```python
from build123d import *

# Parameters (mm, degrees)
BOSS_EXTRUDE1_DEPTH = 9
CUT_EXTRUDE2_REACH  = 95.842
SKETCH5_W           = 20
SKETCH5_H           = 32
SKETCH5_W_2         = 7.75
CUT_EXTRUDE3_DEPTH  = 10
FILLET1_R           = 5
CUT_EXTRUDE4_DEPTH  = 4
CHAMFER1_SIZE       = 9
CHAMFER1_SIZE_2     = 4.196768923
CUT_EXTRUDE5_REACH  = 95.842
SKETCH7_W           = 5
SKETCH7_H           = 33.085129134
SKETCH7_H_2         = 33.745309592


with BuildPart() as part:
    # Sketch1 → Boss-Extrude1 (new body)
    with BuildSketch(Plane(origin=(0, 0, 0), x_dir=(1, 0, 0), z_dir=(0, 1, 0))):
        with BuildLine():
            Line((0, 0), (0, 55))
            Line((0, 55), (75.5, 55))
            Line((75.5, 55), (75.5, 0))
            ThreePointArc((75.5, 0), (37.75, 13.36377481), (0, 0))
        make_face()
    extrude(amount=BOSS_EXTRUDE1_DEPTH)

    # Sketch4 → Cut-Extrude2 (cut, up to next)
    with BuildSketch(Plane(origin=(0, 9, 0), x_dir=(1, 0, 0), z_dir=(0, 1, 0)), mode=Mode.PRIVATE) as cut_extrude2_sk1:
        with BuildLine():
            Line((19.25, 48), (19.25, 23))
            ThreePointArc((19.25, 23), (17.75, 21.5), (16.25, 23))
            Line((16.25, 23), (16.25, 48))
            ThreePointArc((16.25, 48), (17.75, 49.5), (19.25, 48))
        make_face()
    cut_extrude2_tool1 = extrude(cut_extrude2_sk1.sketch, amount=-CUT_EXTRUDE2_REACH, mode=Mode.PRIVATE) & part.part
    # Sketch4 → Cut-Extrude2 (cut, up to next)
    with BuildSketch(Plane(origin=(0, 9, 0), x_dir=(1, 0, 0), z_dir=(0, 1, 0)), mode=Mode.PRIVATE) as cut_extrude2_sk2:
        with BuildLine():
            Line((59.25, 48), (59.25, 23))
            ThreePointArc((59.25, 23), (57.75, 21.5), (56.25, 23))
            Line((56.25, 23), (56.25, 48))
            ThreePointArc((56.25, 48), (57.75, 49.5), (59.25, 48))
        make_face()
    cut_extrude2_tool2 = extrude(cut_extrude2_sk2.sketch, amount=-CUT_EXTRUDE2_REACH, mode=Mode.PRIVATE) & part.part
    add(cut_extrude2_tool1.solids().sort_by_distance((17.75, 9, -35.5))[0], mode=Mode.SUBTRACT)
    add(cut_extrude2_tool2.solids().sort_by_distance((57.75, 9, -35.5))[0], mode=Mode.SUBTRACT)

    # Sketch5 → Cut-Extrude3 (cut)
    with BuildSketch(Plane(origin=(0, 9, 0), x_dir=(1, 0, 0), z_dir=(0, 1, 0))):
        with Locations((37.75, 39)):
            Rectangle(SKETCH5_W, SKETCH5_H)
        with Locations((71.625, 39)):
            Rectangle(SKETCH5_W_2, SKETCH5_H)
        with Locations((3.875, 39)):
            Rectangle(SKETCH5_W_2, SKETCH5_H)
    extrude(amount=-CUT_EXTRUDE3_DEPTH, mode=Mode.SUBTRACT)

    # Fillet1
    fillet1_edges = [part.edges().sort_by_distance(p)[0] for p in [
        (27.75, 4.5, -23),
        (47.75, 4.5, -23),
        (7.75, 4.5, -23),
        (67.75, 4.5, -23),
    ]]
    fillet(fillet1_edges, radius=FILLET1_R)

    # Sketch6 → Cut-Extrude4 (cut)
    with BuildSketch(Plane(origin=(0, 9, 0), x_dir=(1, 0, 0), z_dir=(0, 1, 0))):
        with BuildLine():
            Line((20.55, 48), (20.55, 23))
            ThreePointArc((20.55, 23), (17.75, 20.2), (14.95, 23))
            Line((14.95, 23), (14.95, 48))
            ThreePointArc((14.95, 48), (17.75, 50.8), (20.55, 48))
        make_face()
        with BuildLine():
            Line((60.55, 48), (60.55, 23))
            ThreePointArc((60.55, 23), (57.75, 20.2), (54.95, 23))
            Line((54.95, 23), (54.95, 48))
            ThreePointArc((54.95, 48), (57.75, 50.8), (60.55, 48))
        make_face()
    extrude(amount=-CUT_EXTRUDE4_DEPTH, mode=Mode.SUBTRACT)

    # Chamfer1
    # the kernel refuses this chamfer: 9, 4.196768923 mm, written as the material it takes off along each edge
    with BuildSketch(Plane(origin=(37.75, 9, 46.63622519), x_dir=(0.8768373409785211, 0, -0.4807871436152561), z_dir=(0.4807871436152561, 0, 0.8768373409785211))) as chamfer1_piece_1:
        Polygon((60, -CHAMFER1_SIZE), (60 + CHAMFER1_SIZE_2, 0), (60, 0), align=None)
    revolve(axis=Axis((37.75, 9, 46.63622519), (0, 1, 0)), revolution_arc=122.526351541, mode=Mode.SUBTRACT)

    # Sketch7 → Cut-Extrude5 (cut, up to next)
    with BuildSketch(Plane(origin=(0, 9, 0), x_dir=(1, 0, 0), z_dir=(0, 1, 0)), mode=Mode.PRIVATE) as cut_extrude5_sk1:
        with Locations((2.5, 16.542564567)):
            Rectangle(SKETCH7_W, SKETCH7_H)
    cut_extrude5_tool1 = extrude(cut_extrude5_sk1.sketch, amount=-CUT_EXTRUDE5_REACH, mode=Mode.PRIVATE) & part.part
    # Sketch7 → Cut-Extrude5 (cut, up to next)
    with BuildSketch(Plane(origin=(0, 9, 0), x_dir=(1, 0, 0), z_dir=(0, 1, 0)), mode=Mode.PRIVATE) as cut_extrude5_sk2:
        with Locations((73, 16.872654796)):
            Rectangle(SKETCH7_W, SKETCH7_H_2)
    cut_extrude5_tool2 = extrude(cut_extrude5_sk2.sketch, amount=-CUT_EXTRUDE5_REACH, mode=Mode.PRIVATE) & part.part
    add(cut_extrude5_tool1.solids().sort_by_distance((2.5, 9, -16.542565))[0], mode=Mode.SUBTRACT)
    add(cut_extrude5_tool2.solids().sort_by_distance((73, 9, -16.872655))[0], mode=Mode.SUBTRACT)


solid = part.part
```
Design review of the part built by this model. Coordinates are the model's own, in mm. A direction names the side the tool comes from. Coordinates: 2 decimals unless noted, no trailing zeros. Order: outer loops, then holes, each group sorted by start corner. A loop starts at its lowest first (then second) coordinate and runs counter-clockwise, first axis right, second up.
1) Take a section at B-B, the plane y = 2.75. Give the boundary of the cut face in (x, z), and give its area (3 significant figures).
2) Wall thickness on line 1 along X through (y, z) = (3.75, -31); line 2 along X through (y, z) = (5.75, -20.5); line 3 along X through (y, z) = (2, -49): over which ranges is each line inside the solid? List them lowest first.
3) Mouldability with a two-part tool opening along X and no side actions: class faces 6 (the flat face through (7.75, 5, -41)), 7 (the cylindrical face through (57.7, 7, -50.8)), 8 (the flat face through (18, 4, -55)), 9 (the flat face through (67.75, 5, -41)) as +X half, -X half, draft (parallel to the pull), parting line (faces both ways), or undercut.
4) Take a section at C-C, the plane y = 6. Give the boundary of the cut face in (x, z).
5) For faces 1 (the conical face through (38.25, 3.56, -15.02)), 2 (the flat face through (47.75, 5, -41)), 3 (the cylindrical face through (17.7, 2.5, -49.5)), 4 (the flat face through (58, 4, -55)), 5 (the cylindrical face through (17.7, 7, -50.8)), list the 3-axis set-ups (+Z, -Z, +X, -X, +Y, -Y) from which the entire face can be reached by the end or side of a thin tool; tool diameter is ignored.
6) Clearance check with flat-ended pins moving along their axes: pin 1 (3 mm diameter, centred on y = 7.5, z = -35.5, fed in from +X); pin 2 (1.2 mm diameter, centred on y = 6, z = -36.5, fed in from -X); pin 3 (1 mm diameter, centred on x = 27, y = 7, fed in from +Z). State where each tip first meets the part, or that it passes through.
7) Take a section at A-A, the plane z = -35.5. Give the boundary of the cut face in (x, y).
Returned:
1. outline: (5, -23.53) arc R5 cw to (7.75, -28) - (7.75, -55) - (27.75, -55) - (27.75, -28) arc R5 cw to (32.75, -23) - (42.75, -23) arc R5 cw to (47.75, -28) - (47.75, -55) - (67.75, -55) - (67.75, -28) arc R5 cw to (70.5, -23.53) - (70.5, -5.16) arc R61.28 cw to (5, -5.16) - close; hole (16.25, -48) arc R1.5 ccw to (19.25, -48) - (19.25, -23) arc R1.5 ccw to (16.25, -23) - close; hole (56.25, -48) arc R1.5 ccw to (59.25, -48) - (59.25, -23) arc R1.5 ccw to (56.25, -23) - close
1. area: 1,880 mm2
2. line 1: x = 7.75 to 16.25, 19.25 to 27.75, 47.75 to 56.25, 59.25 to 67.75
2. line 2: x = 5 to 16.49, 19.01 to 56.49, 59.01 to 70.5
2. line 3: x = 7.75 to 16.63, 18.87 to 27.75, 47.75 to 56.63, 58.87 to 67.75
3. face 6: -X half
3. face 7: undercut
3. face 8: draft
3. face 9: +X half
4. outline: (5, -23.53) arc R5 cw to (7.75, -28) - (7.75, -55) - (27.75, -55) - (27.75, -28) arc R5 cw to (32.75, -23) - (42.75, -23) arc R5 cw to (47.75, -28) - (47.75, -55) - (67.75, -55) - (67.75, -28) arc R5 cw to (70.5, -23.53) - (70.5, -6.95) arc R62.8 cw to (5, -6.95) - close; hole (14.95, -48) arc R2.8 ccw to (20.55, -48) - (20.55, -23) arc R2.8 ccw to (14.95, -23) - close; hole (54.95, -48) arc R2.8 ccw to (60.55, -48) - (60.55, -23) arc R2.8 ccw to (54.95, -23) - close
5. face 1: +Z, +Y
5. face 2: -Z, +Y, -Y
5. face 3: +Y, -Y
5. face 4: -Z, +X, -X, +Y, -Y
5. face 5: +Y
6. pin 1: stops at x = 67.75
6. pin 2: stops at x = 7.75
6. pin 3: stops at z = -15.46
7. outline: (7.75, 0) - (16.25, 0) - (16.25, 5) - (14.95, 5) - (14.95, 9) - (7.75, 9) - close; (19.25, 0) - (27.75, 0) - (27.75, 9) - (20.55, 9) - (20.55, 5) - (19.25, 5) - close; (47.75, 0) - (56.25, 0) - (56.25, 5) - (54.95, 5) - (54.95, 9) - (47.75, 9) - close; (59.25, 0) - (67.75, 0) - (67.75, 9) - (60.55, 9) - (60.55, 5) - (59.25, 5) - close
